Study the drawing (mm; zero at the part's minimum x, y, z) and answer. Coordinates: 2 decimals unless noted, no trailing zeros. Order: outer loops, then holes, each group sorted by start corner. A loop starts at its lowest first (then second) coordinate and runs counter-clockwise, first axis right, second up.
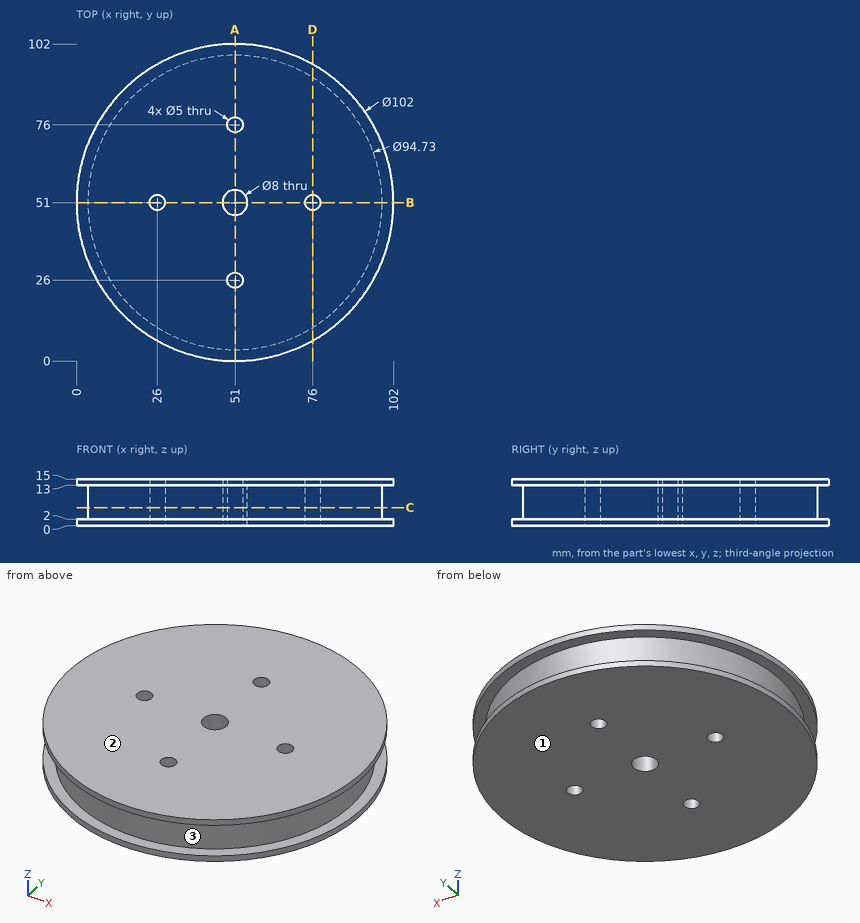
1) Flat-ended cylindrical pins translate along their axes: pin 1 Ø4 at (y, z) = (79, 7.5) entering from +X; pin 2 Ø3 at (y, z) = (84, 4.5) entering from +X; pin 3 Ø1 at (y, z) = (78.5, 9) entering from -X. Find the tip coordinate at first contact, or state that the pin passes through.
A:
pin 1: stops at x = 90.59
pin 2: stops at x = 86.37
pin 3: stops at x = 12.08
2) A cutting plane is placed at A-A, the plane x = 51. Determine the outline of the cut face in (y, z) (3 decimals).
A:
outline: (0, 0) - (23.5, 0) - (23.5, 15) - (0, 15) - (0, 13) - (3.635, 13) - (3.635, 2) - (0, 2) - close; (28.5, 0) - (47, 0) - (47, 15) - (28.5, 15) - close; (55, 0) - (73.5, 0) - (73.5, 15) - (55, 15) - close; (78.5, 0) - (102, 0) - (102, 2) - (98.365, 2) - (98.365, 13) - (102, 13) - (102, 15) - (78.5, 15) - close
3) Straight lines are drawn through the part: line 1 (Y direction, x = 51, z = 3.5) (3 decimals); line 2 (X direction, y = 25, z = 5.25); line 3 (Y direction, x = 54.5, z = 11.25). For each, find the intervals that lie inside material, in ascending order.
A:
line 1: y = 3.635 to 23.5, 28.5 to 47, 55 to 73.5, 78.5 to 98.365
line 2: x = 11.41 to 48.71, 53.29 to 90.59
line 3: y = 3.76 to 49.06, 52.94 to 98.24
4) A cutting plane is placed at D-D, the plane x = 76. Determine the outline of the cut face in (y, z), and give its area (3 significant figures).
A:
outline: (6.55, 0) - (48.5, 0) - (48.5, 15) - (6.55, 15) - (6.55, 13) - (10.77, 13) - (10.77, 2) - (6.55, 2) - close; (53.5, 0) - (95.45, 0) - (95.45, 2) - (91.23, 2) - (91.23, 13) - (95.45, 13) - (95.45, 15) - (53.5, 15) - close
area: 1,170 mm2
5) A cutting plane is placed at C-C, the plane z = 5.75. Determine the outline of the cut face in (x, y) (3 decimals).
A:
outline: circle Ø94.73 at (51, 51); hole circle Ø5 at (26, 51); hole circle Ø8 at (51, 51); hole circle Ø5 at (51, 26); hole circle Ø5 at (51, 76); hole circle Ø5 at (76, 51)
6) Determine the mould class of the marked faces 1, 2 and 3 for opening direction Z: pulls with the +Z half, pulls with the -Z half, needs draft (parallel to the pull), parting line crosses it, or undercut.
A:
face 1: pulls with the -Z half
face 2: pulls with the +Z half
face 3: undercut
